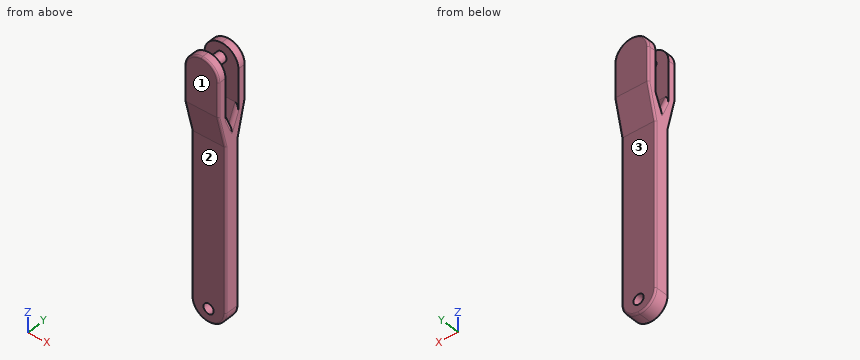
```python
from build123d import *

# Parameters (mm, degrees)
BOSS_EXTRUDE1_DEPTH     = 50
CUT_EXTRUDE1_DEPTH      = 745.983221288
CUT_EXTRUDE1_DEPTH_BACK = 745.983221288
SKETCH3_R               = 15
SKETCH4_R               = 15
BOSS_EXTRUDE2_DEPTH     = 95
FILLET1_R               = 50
FILLET2_R               = 10
FILLET3_R               = 50
FILLET4_R               = 5


with BuildPart() as part:
    # Sketch2 → Boss-Extrude1 (new, symmetric)
    with BuildSketch(Plane(origin=(0, 0, 0), x_dir=(0, 0, -1), z_dir=(1, 0, 0))):
        Polygon((0, -22.5), (40, -22.5), (40, 22.5), (0, 22.5), (-490, 22.5), (-590, 47.5), (-740, 47.5), (-740, 22.5), (-590, 22.5), (-540, 0), (-590, -22.5), (-740, -22.5), (-740, -47.5), (-590, -47.5), (-490, -22.5), align=None)
    extrude(amount=BOSS_EXTRUDE1_DEPTH, both=True)

    # Sketch3 → Cut-Extrude1 (cut, two sides: drawn at the far end of the back side and taken through both)
    with BuildSketch(Plane.XZ.offset(22.5).offset(-CUT_EXTRUDE1_DEPTH_BACK)):
        with Locations(Location((0, 0, 0), (0, 0, 270))):
            Circle(SKETCH3_R)
    extrude(amount=CUT_EXTRUDE1_DEPTH + CUT_EXTRUDE1_DEPTH_BACK, mode=Mode.SUBTRACT)

    # Sketch4 → Boss-Extrude2 (add)
    with BuildSketch(Plane.XZ.offset(47.5)):
        with Locations(Location((0, 700, 0), (0, 0, 270))):
            Circle(SKETCH4_R)
    extrude(amount=-BOSS_EXTRUDE2_DEPTH)

    # Fillet1
    fillet1_edges = [part.edges().sort_by_distance(p)[0] for p in [
        (50, 0, -40),
        (-50, 0, -40),
    ]]
    fillet(fillet1_edges, radius=FILLET1_R - 0.0001)  # a hair under: the kernel refuses the full size

    # Fillet2
    fillet2_edges = [part.edges().sort_by_distance(p)[0] for p in [
        (-50, -11.25, 565),
        (-50, 11.25, 565),
        (50, 11.25, 565),
        (50, -11.25, 565),
    ]]
    fillet(fillet2_edges, radius=FILLET2_R)

    # Fillet3
    fillet3_edges = [part.edges().sort_by_distance(p)[0] for p in [
        (-50, -35, 740),
        (-50, 35, 740),
        (50, 35, 740),
        (50, -35, 740),
    ]]
    fillet(fillet3_edges, radius=FILLET3_R - 0.0001)  # a hair under: the kernel refuses the full size

    # Fillet4
    fillet4_edges = [part.edges().sort_by_distance(p)[0] for p in [
        (-50, -47.5, 640.00005),
        (50, -47.5, 640.00005),
        (35.355368349, -47.5, 725.355368349),
        (-35.355368349, -47.5, 725.355368349),
        (35.355368349, 47.5, 725.355368349),
        (-35.355368349, 47.5, 725.355368349),
        (-50, -35, 540),
        (-50, 47.5, 640.00005),
        (-50, 35, 540),
        (-50, -22.5, 249.99995),
        (50, 35, 540),
        (50, 47.5, 640.00005),
        (50, -22.5, 249.99995),
        (50, 22.5, 249.99995),
        (50, -35, 540),
        (-50, 22.5, 249.99995),
        (-35.355368349, 22.5, -25.355368349),
        (35.355368349, 22.5, -25.355368349),
        (-35.355368349, -22.5, -25.355368349),
        (35.355368349, -22.5, -25.355368349),
    ]]
    fillet(fillet4_edges, radius=FILLET4_R)


solid = part.part
```
Read the model definition and answer for the solid it produces. Units are mm, in the model's axes. Face numbers are marked on the shaded views. A direction names the side the tool comes from. Coordinates: 2 decimals unless noted, no trailing zeros. Loops run counter-clockwise (first coordinate to the right, second up) from the corner with the lowest first, then second, coordinate; pieces in that order, holes last. Notation, with made-up numbers: (30.5, 71.5) -> (39.5, 71.5) arc R10 cw to (39.5, 75.5) -> close; hole circle Ø5 at (32.5, 81). An arc over 180 degrees is marked (long way). Return JSON: item names as keys, results as strings.
Item 1: Find section C-C (y = 6.5). Count the separate pieces of the cut face and the enclosed holes in it, plus the area to 3 significant figures.
Answers:
{"separate pieces": "2", "enclosed holes": "1", "area": "58,300 mm2"}
Item 2: For the marked faces 1, 2 and 3, determine the directions among +Z, -Z, +X, -X, +Y, -Y from which every point of the face is accessible in a straight line to the end or side of a thin tool.
Answers:
{"face 1": "+Z, -Z, +X, -X, -Y", "face 2": "-Z, +X, -X, -Y", "face 3": "-Z, +X, -X, +Y"}
Item 3: Find the intervals of material crossed by probe 1 along Y at (x, z) = (12, 632); probe 2 along Y at (x, z) = (-35, 334.5); probe 3 along X at (y, z) = (-18.5, 358), in increasing order.
Answers:
{"probe 1": "y = -47.5 to -22.5, 22.5 to 47.5", "probe 2": "y = -22.5 to 22.5", "probe 3": "x = -49.9 to 49.9"}
Item 4: Find section B-B (z = 198). Determine the outline of the cut face in (x, y).
Answers:
{"outline": "(-50, -17.5) arc R5 ccw to (-45, -22.5) -> (45, -22.5) arc R5 ccw to (50, -17.5) -> (50, 17.5) arc R5 ccw to (45, 22.5) -> (-45, 22.5) arc R5 ccw to (-50, 17.5) -> close"}
Item 5: Find section A-A (z = 646.5). Determine the outline of the cut face in (x, y).
Answers:
{"outline": "(-50, -42.5) arc R5 ccw to (-45, -47.5) -> (45, -47.5) arc R5 ccw to (50, -42.5) -> (50, -22.5) -> (-50, -22.5) -> close; (-50, 22.5) -> (50, 22.5) -> (50, 42.5) arc R5 ccw to (45, 47.5) -> (-45, 47.5) arc R5 ccw to (-50, 42.5) -> close"}
Item 6: Flat-ended cylindrical pins translate along their axes: P1, Ø10, axis at x = 19, y = 7, coming from the -Z side; P2, Ø1, axis at x = -21, y = -13.5, coming from the +Z side; P3, Ø1, axis at x = -22, y = -26, coming from the +Z side. Find the tip coordinate at first contact, or state that the pin passes through.
Answers:
{"P1": "stops at z = -38", "P2": "stops at z = 571.11", "P3": "stops at z = 735.14"}
